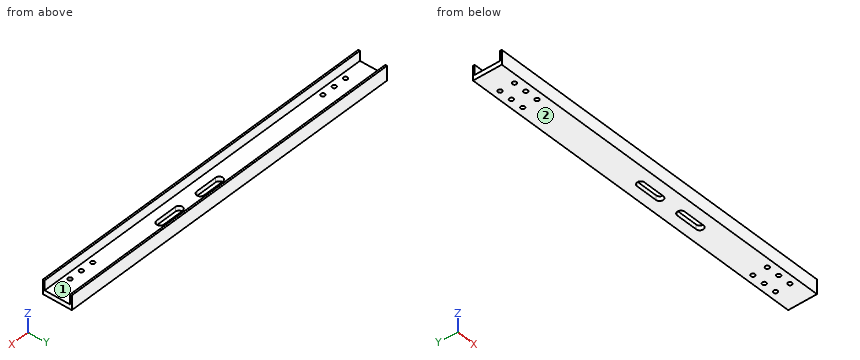
```python
from build123d import *

# Parameters (mm, degrees)
SKETCH1_W               = 34
SKETCH1_H               = 6
SKETCH1_W_2             = 16
SKETCH1_H_2             = 88
BOSS_EXTRUDE1_DEPTH     = 1254
F_12_0MM_DOWEL_HOLE1_D  = 14
CUT_EXTRUDE1_DEPTH      = 35
CUT_EXTRUDE1_DEPTH_BACK = 17


with BuildPart() as part:
    # Sketch1 → Boss-Extrude1 (new body)
    with BuildSketch(Plane(origin=(0, 0, 0), x_dir=(0, 0, -1), z_dir=(1, 0, 0))):
        with Locations((-25, 47)):
            Rectangle(SKETCH1_W, SKETCH1_H)
        with Locations((0, 47)):
            Rectangle(SKETCH1_W_2, SKETCH1_H)
        Rectangle(SKETCH1_W_2, SKETCH1_H_2)
        with Locations((0, -47)):
            Rectangle(SKETCH1_W_2, SKETCH1_H)
        with Locations((-25, -47)):
            Rectangle(SKETCH1_W, SKETCH1_H)
    extrude(amount=BOSS_EXTRUDE1_DEPTH)

    # Ø12.0mm Dowel Hole1 (through all)
    with Locations(Plane.XY.offset(8)):
        with Locations((1175, 25), (1130, 25), (1085, 25), (1085, -25), (1130, -25), (1175, -25), (79, 25), (124, 25), (169, 25), (169, -25), (124, -25), (79, -25)):
            Hole(F_12_0MM_DOWEL_HOLE1_D / 2)

    # Sketch7 → Cut-Extrude1 (cut, two sides)
    with BuildSketch(Plane.XY.offset(8)) as cut_extrude1_sk:
        with BuildLine():
            Line((770.18, 12.5), (845.18, 12.5))
            ThreePointArc((845.18, 12.5), (857.68, 0), (845.18, -12.5))
            Line((845.18, -12.5), (770.18, -12.5))
            ThreePointArc((770.18, -12.5), (757.68, 0), (770.18, 12.5))
        make_face()
        with BuildLine():
            Line((685.18, -12.5), (610.18, -12.5))
            ThreePointArc((610.18, -12.5), (597.68, 0), (610.18, 12.5))
            Line((610.18, 12.5), (685.18, 12.5))
            ThreePointArc((685.18, 12.5), (697.68, 0), (685.18, -12.5))
        make_face()
    extrude(amount=CUT_EXTRUDE1_DEPTH, mode=Mode.SUBTRACT)
    extrude(cut_extrude1_sk.sketch, amount=-CUT_EXTRUDE1_DEPTH_BACK, mode=Mode.SUBTRACT)


solid = part.part
```
Can you work these out from the model? Positions are in its coordinate system, mm. Face numbers are marked on the shaded views. A direction names the side the tool comes from. Give positions to 0.01 mm unless a question says otherwise; leave off trailing zeros. Write each loop counter-clockwise with the first axis right and the second up, starting at its lowest first coordinate (ties: lowest second). Pieces come first, ordered by that corner, then holes. Notation, with made-up numbers: (23, 76) -> (58, 76) arc R22 cw to (58, 97) -> close; hole circle Ø10 at (82.5, -0.75). An arc over 180 degrees is marked (long way). Write item = value, one per line.
(1) For the marked faces 1 and 2, which set-ups out of +Z, -Z, +X, -X, +Y, -Y let a thin tool reach every point of the face, with its end or its side?
Worked out:
face_1 = +Z, +X, -X
face_2 = -Z, +X, -X, +Y, -Y
(2) I'm going to push flat-ended pins straight in: P1, Ø22.5, axis at x = 124, y = -25, coming from the -Z side; P2, Ø3, axis at x = 696.5, y = -39.5, coming from the +Z side. Where does each tip first touch, or does it pass through?
Worked out:
P1 = -8
P2 = 8
(3) I need wall thicknesses on probe 1 along Y at (x, z) = (79, -1.25); probe 2 along Y at (x, z) = (536.5, 22); probe 3 along Z at (x, y) = (404, 36). Which ranges of each line are inside material? Lowest first, please. Write a range as from..to.
Worked out:
probe_1 = -50..-32, -18..18, 32..50
probe_2 = -50..-44, 44..50
probe_3 = -8..8
(4) Suppose I cut it at B-B on z = 28. Write out the boundary of the cut face in (x, y), then the cut area to 3 significant figures.
Worked out:
outline = (0, -50) -> (1254, -50) -> (1254, -44) -> (0, -44) -> close; (0, 44) -> (1254, 44) -> (1254, 50) -> (0, 50) -> close
area = 15,000 mm^2
(5) Suppose I cut it at A-A on x = 623. Write out the boundary of the cut face in (y, z).
Worked out:
outline = (-50, -8) -> (-12.5, -8) -> (-12.5, 8) -> (-44, 8) -> (-44, 42) -> (-50, 42) -> close; (12.5, -8) -> (50, -8) -> (50, 42) -> (44, 42) -> (44, 8) -> (12.5, 8) -> close
